Verification items for the finished model (mm, model axes). Coordinates: 2 decimals unless noted, no trailing zeros. Order: outer loops, then holes, each group sorted by start corner. A loop starts at its lowest first (then second) coordinate and runs counter-clockwise, first axis right, second up. Notation, with made-up numbers: (76.25, 42) -> (103.25, 42) arc R23 ccw to (103.25, 69) -> close; hole circle Ø10 at (12, -32). An arc over 180 degrees is marked (long way). Write item = value, one per line. Start each with the question number.
1. Cross-section at A-A on y = 0.5. Record the cut outline in (x, z).
2. Cross-section at B-B on x = -15.5. Record the cut outline in (y, z).
3. Cross-section at C-C on z = -503.5. Record the cut outline in (x, y).
4. Thickness scan on line 1 along Z through (x, y) = (5.5, 5); line 2 along Z through (x, y) = (3, 16); line 3 along Z through (x, y) = (-15, 14.5). Record the ranges inside material, lowest first. Write a range as from..to.
5. Go/stop test with flat-tipped pins: P1, Ø8, axis at x = -15.5, y = 8.5, coming from the -Z side; P2, Ø6, axis at x = 11.5, y = 3, coming from the +Z side; P3, Ø2, axis at x = 17, y = -12.5, coming from the +Z side; P4, Ø22.5, axis at x = -2.5, z = 672, coming from the -Y side. Record where each tip stops, or that it passes through.
from build123d import *

# Parameters (mm, degrees)
F0_W      = 45
F0_H      = 45
F1_DEPTH  = 650
F3_DEPTH  = 14
F4_W      = 16
F4_H      = 45
F5_DEPTH  = 45.001
F6_W      = 18
F6_H      = 45
F7_DEPTH  = 45.001
F8_W      = 16
F8_H      = 45
F9_DEPTH  = 45.001
F10_W     = 45
F10_H     = 17
F11_DEPTH = 63.6
F13_DEPTH = 31.001


# Not quite as in the source:
# - a pattern or mirror of a feature is missing from the dataset's text; its kind, count and spacing are read off the source's solid


with BuildPart() as f1:
    # F0 (on Top) → F1 (new body, symmetric)
    with BuildSketch(Plane.XY):
        Rectangle(F0_W, F0_H)
    extrude(amount=F1_DEPTH, both=True)

    # F2 (on face) → F3 (cut)
    with BuildSketch(Plane.XZ.offset(22.5)):
        Polygon((22.5, 650), (0, 650), (22.5, 627.5), align=None)
        Polygon((-22.5, 627.5), (0, 650), (-22.5, 650), align=None)
    f3 = extrude(amount=-F3_DEPTH, mode=Mode.SUBTRACT)

    # F3_copies: F3 across plane
    add(f3.mirror(Plane.ZX), mode=Mode.SUBTRACT)

    # F4 (on face) → F5 (cut, through all)
    with BuildSketch(Plane.XZ.offset(22.5)):
        with Locations((0, -500)):
            Rectangle(F4_W, F4_H)
    extrude(amount=-F5_DEPTH, mode=Mode.SUBTRACT)

    # F6 (on face) → F7 (cut, through all)
    with BuildSketch(Plane.YZ.offset(22.5)):
        with Locations((0, -627.5)):
            Rectangle(F6_W, F6_H)
    extrude(amount=-F7_DEPTH, mode=Mode.SUBTRACT)

    # F8 (on face) → F9 (cut, through all)
    with BuildSketch(Plane.XZ.offset(22.5)):
        with Locations((0, 377.5)):
            Rectangle(F8_W, F8_H)
    extrude(amount=-F9_DEPTH, mode=Mode.SUBTRACT)

    # F10 (on face) → F11 (join)
    with BuildSketch(Plane.XY.offset(650)):
        Rectangle(F10_W, F10_H)
    extrude(amount=F11_DEPTH)

    # F12 (on face) → F13 (cut, through all)
    with BuildSketch(Plane.XZ.offset(8.5)):
        Polygon((-22.5, 691.1), (0, 713.6), (-22.5, 713.6), align=None)
        Polygon((22.5, 713.6), (0, 713.6), (22.5, 691.1), align=None)
    extrude(amount=-F13_DEPTH, mode=Mode.SUBTRACT)


solid = f1.part
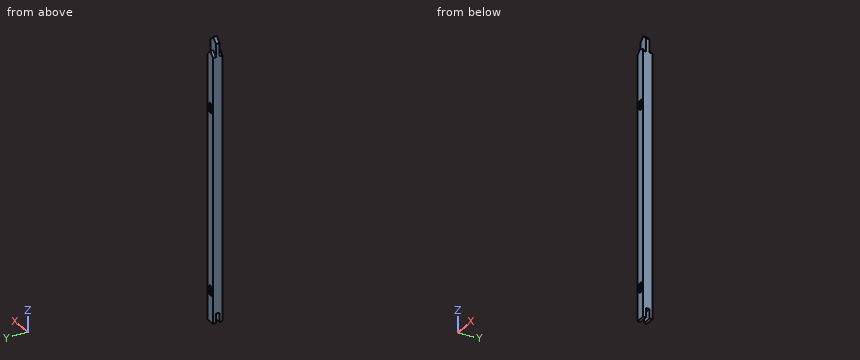
Worked out:
q1.outline = (-22.5, -605) -> (22.5, -605) -> (22.5, 691.1) -> (0, 713.6) -> (-22.5, 691.1) -> close; hole (-8, -522.5) -> (8, -522.5) -> (8, -477.5) -> (-8, -477.5) -> close; hole (-8, 355) -> (8, 355) -> (8, 400) -> (-8, 400) -> close
q2.outline = (-22.5, -650) -> (-9, -650) -> (-9, -605) -> (9, -605) -> (9, -650) -> (22.5, -650) -> (22.5, 634.5) -> (8.5, 634.5) -> (8.5, 698.1) -> (-8.5, 698.1) -> (-8.5, 634.5) -> (-22.5, 634.5) -> close
q3.outline = (-22.5, -22.5) -> (-8, -22.5) -> (-8, 22.5) -> (-22.5, 22.5) -> close; (8, -22.5) -> (22.5, -22.5) -> (22.5, 22.5) -> (8, 22.5) -> close
q4.line_1 = -605..-522.5, -477.5..355, 400..708.1
q4.line_2 = -650..-522.5, -477.5..355, 400..647
q4.line_3 = -650..635
q5.P1 = -650
q5.P2 = 705.1
q5.P3 = 634
q5.P4 = -8.5
